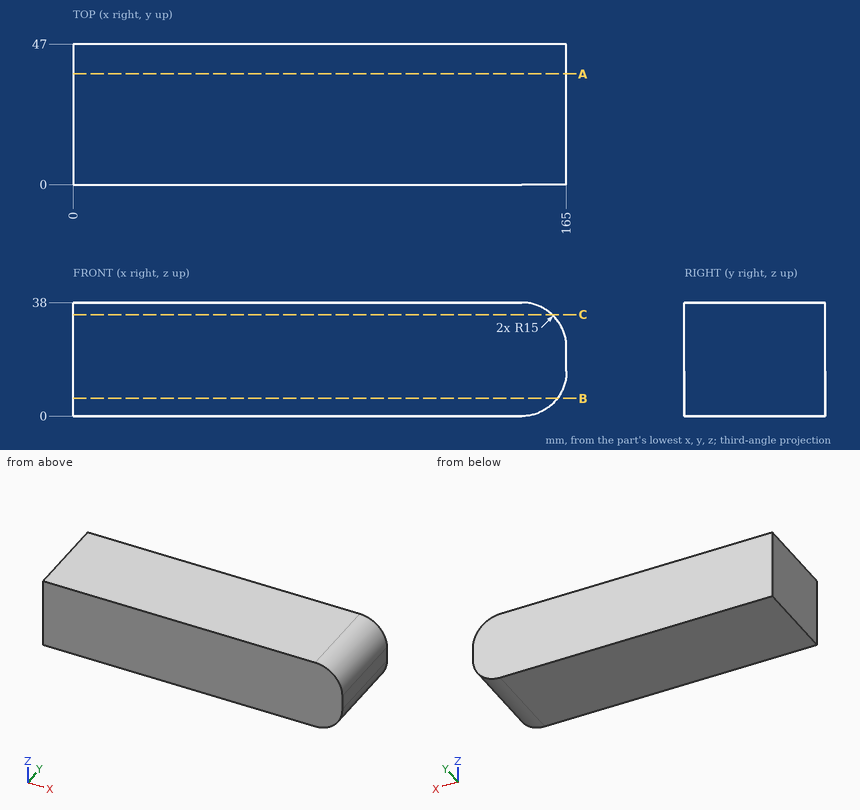
Geometry: see drawing. Coordinates: mm, zero at the bounding-box minimum. Give positions to 0.01 mm unless a question says otherwise; leave off trailing zeros. Write each loop counter-clockwise with the first axis right and the second up, starting at its lowest first coordinate (ties: lowest second). Pieces come first, ordered by that corner, then holes. Notation, with made-up numbers: (-29, 46) - (6, 46) arc R14 cw to (6, 56) - close; hole circle Ø10 at (23.5, -39). An arc over 180 degrees is marked (long way). Return JSON: item names as keys, results as strings. Group by question number.
1) Section B-B on z = 6. Return the cut outline in (x, y).
2) Line query: line 1 (X direction, y = 14, z = 27); line 2 (X direction, y = 34, z = 29). Output: solid intervals per line, ascending.
3) Section A-A on y = 37. Return the cut outline in (x, z).
4) Section C-C on z = 34. Return the cut outline in (x, y).
Filled in:
{
 "1": {"outline": "(0, 0) - (162, 0) - (162, 47) - (0, 47) - close"},
 "2": {"line 1": "x = 0 to 164.46", "line 2": "x = 0 to 163.75"},
 "3": {"outline": "(0, 0) - (150, 0) arc R15 ccw to (165, 15) - (165, 23) arc R15 ccw to (150, 38) - (0, 38) - close"},
 "4": {"outline": "(0, 0) - (160.2, 0) - (160.2, 47) - (0, 47) - close"}
}
